Here's how the part is built. I have some questions about the finished solid (model axes, mm). Round coordinates to 2 decimals unless told otherwise and drop trailing zeros. Write each loop counter-clockwise with the first axis right and the second up, starting at its lowest first coordinate (ties: lowest second). Pieces come first, ordered by that corner, then holes. Notation, with made-up numbers: (89, 42) - (145, 42) arc R18 cw to (145, 54) - close; hole circle Ø8 at (-35.75, -33.5). An arc over 180 degrees is marked (long way). One line per item, written item: value. Start each with the question number.
Item 1: If I drill on line 1 (Y direction, x = 8.75, z = 343.5); line 2 (Z direction, x = 4.25, y = -30); line 3 (Z direction, x = 6.25, y = -21.5), over which ranges is the centre line in solid material (lowest first)?
Item 2: Imagine slicing it at A-A, the plane z = 271.5. Please give me the cut outline in (x, y), then the cut area to 3 significant figures.
Item 3: For P1, Ø1.5, axis at x = 7, y = -37, coming from the -Z side (3 decimals); P2, Ø7.5, axis at x = -2, z = 24, coming from the -Y side; P3, Ø4, axis at x = -2.5, y = -40.5, coming from the -Z side; P4, Ø10, axis at x = 9.5, y = -9.5, coming from the +Z side, each with a flat end and sliding along its axis, tell me the tip position at first contact or that it passes through.
Item 4: Imagine slicing it at B-B, the plane y = -39.5. Please give me the cut outline in (x, z), then the cut area to 3 significant figures.
Item 5: Thinking about a two-plate mould opening in Z: for faces 1 (the face through (0, -25, 6)), 2 (the face through (-8.935, -12.675, -396.241)), 3 (the face through (-12.5, -12, -5)), which applies, released by +Z, released by -Z, zero draft, split by the parting line, or undercut?
```python
from build123d import *

# Parameters (mm, degrees)
F0_W     = 25
F0_H     = 800
F1_DEPTH = 25
F2_R     = 5
F3_DEPTH = 25
F4_R     = 5
F5_DEPTH = 25
F6_R     = 12.49999
F7_R     = 12.49999


# Not quite as in the source:
# - a fillet or chamfer is up to 0.001 mm smaller than in the source, because OpenCascade refuses the exact size
# - a pattern or mirror of a feature is missing from the dataset's text; its kind, count and spacing are read off the source's solid


with BuildPart() as f1:
    # F0 (on Front) → F1 (new body)
    with BuildSketch(Plane.XZ):
        Rectangle(F0_W, F0_H)
    extrude(amount=F1_DEPTH)

    # F2 (on face) → F3 (join)
    with BuildSketch(Plane.XZ.offset(25)):
        with Locations((0, 391.8639719486)):
            Circle(F2_R)
    f3 = extrude(amount=F3_DEPTH)

    # F3_copies: F3 across plane
    add(f3.mirror(Plane(origin=(0, 0, 0), x_dir=(-1, 0, 0), z_dir=(0, 0, -1))))

    # F4 (on face) → F5 (cut)
    with BuildSketch(Plane.XZ.offset(25)):
        Circle(F4_R)
    extrude(amount=-F5_DEPTH, mode=Mode.SUBTRACT)

    # F6 (radius 12.5 in the source; OpenCascade refuses exactly that, so slightly less here)
    f6_edges = [f1.edges().sort_by_distance(p)[0] for p in [
        (-12.5, -12.5, 400),
        (12.5, -12.5, 400),
    ]]
    fillet(f6_edges, radius=F6_R)

    # F7 (radius 12.5 in the source; OpenCascade refuses exactly that, so slightly less here)
    f7_edges = [f1.edges().sort_by_distance(p)[0] for p in [
        (12.5, -12.5, -400),
        (-12.5, -12.5, -400),
    ]]
    fillet(f7_edges, radius=F7_R)


solid = f1.part
```
Values follow:
1. line 1: y = -25 to 0
1. line 2: z = -394.5 to -389.23, 389.23 to 394.5
1. line 3: z = -398.33 to 398.33
2. outline: (-12.5, -25) - (12.5, -25) - (12.5, 0) - (-12.5, 0) - close
2. area: 625 mm^2
3. P1: passes through
3. P2: stops at y = -25
3. P3: stops at z = -396.84
3. P4: stops at z = 399.16
4. outline: circle Ø10 at (0, -391.86); circle Ø10 at (0, 391.86)
4. area: 157 mm^2
5. face 1: undercut
5. face 2: released by -Z
5. face 3: zero draft
